Input: dimensioned drawing with shaded views. Units: mm. Origin: part minimum x, y, z. A direction names the side the tool comes from. Coordinates: 2 decimals unless noted, no trailing zeros. Write each loop counter-clockwise with the first axis right and the second up, starting at its lowest first coordinate (ties: lowest second). Pieces come first, ordered by that corner, then holes. Notation, with made-up numbers: (84.25, 32) -> (93.25, 32) arc R26 cw to (93.25, 56) -> close; hole circle Ø10 at (-19, 36). An arc over 180 degrees is marked (long way). One line per item, written item: value. Start each with the question number.
1. Access query for the marked faces 1 and 2. Directions: +Z, -Z, +X, -X, +Y, -Y. A direction counts if a zero-diameter tool reaches every point of the face in a straight line with its end or side. Return the directions, or none.
2. Section query C-C, the plane z = 3.75. Output: boundary loops of the cut face in (x, y), and give its area (3 significant figures).
3. Section query D-D, the plane y = 7. Output: boundary loops of the cut face in (x, z) (1 decimal).
4. First-contact query: P1, Ø3, axis at y = 3, z = 2, coming from the +X side; P2, Ø1, axis at y = 13, z = 8, coming from the +X side; P3, Ø3, axis at y = 10.5, z = 3, coming from the +X side (1 decimal); P4, Ø10, axis at x = 8.5, z = 14.5, coming from the +Y side. Flat tips, straight axial feed; report the tip coordinate or a pass-through.
5. Line query: line 1 (Z direction, x = 12, y = 14) (1 decimal); line 2 (Z direction, x = 9, y = 3.5) (1 decimal); line 3 (Y direction, x = 11, z = 27.5). Output: solid intervals per line, ascending.
6. Section query B-B, the plane z = 21.5. Output: boundary loops of the cut face in (x, y), and give its area (3 significant figures).
7. Section query A-A, the plane y = 20.32. Output: boundary loops of the cut face in (x, z) (1 decimal).
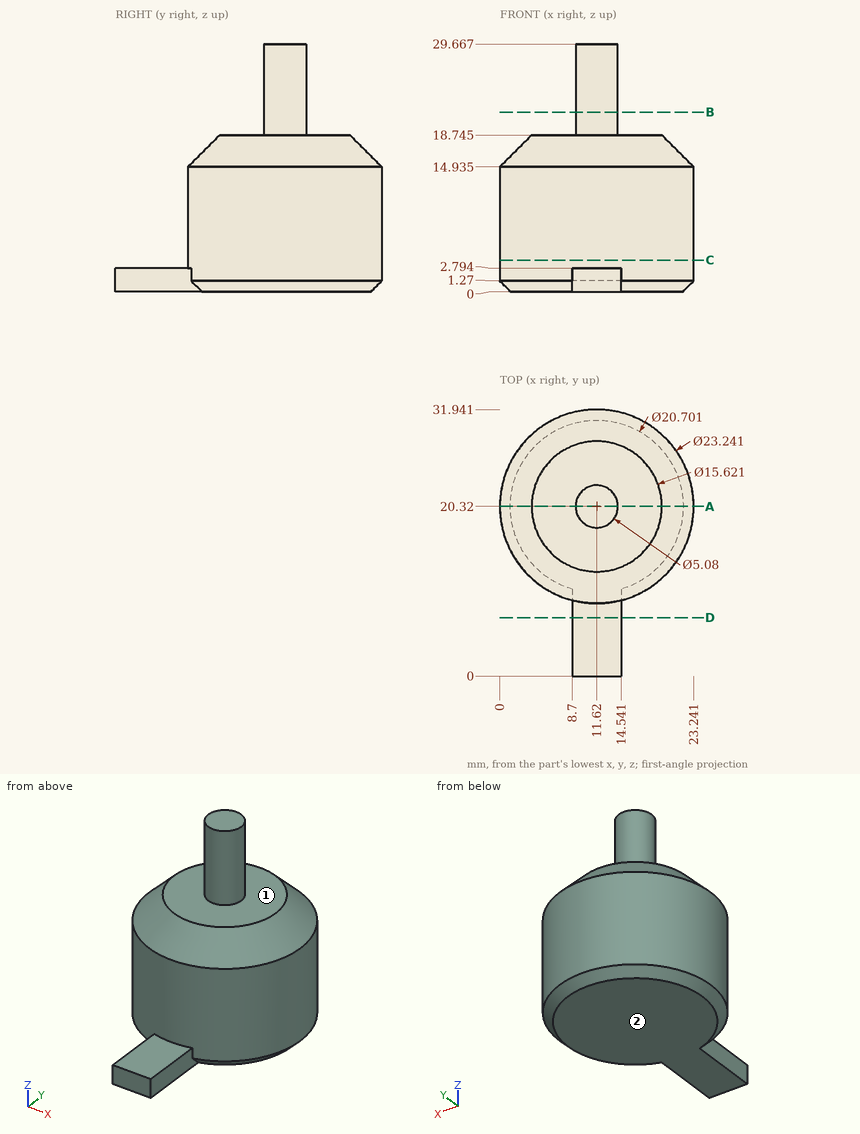
Computed values:
1. face 1: +Z
1. face 2: -Z, +X, -X, +Y, -Y
2. outline: circle Ø23.24 at (11.62, 20.32)
2. area: 424 mm²
3. outline: (8.7, 0) -> (14.5, 0) -> (14.5, 2.8) -> (8.7, 2.8) -> close
4. P1: stops at x = 14.54
4. P2: stops at x = 21.03
4. P3: stops at x = 19.7
4. P4: stops at y = 31.94
5. line 1: z = 0 to 18.7
5. line 2: z = 0 to 2.8
5. line 3: y = 17.86 to 22.78
6. outline: circle Ø5.08 at (11.62, 20.32)
6. area: 20.3 mm²
7. outline: (0, 1.3) -> (1.3, 0) -> (22, 0) -> (23.2, 1.3) -> (23.2, 14.9) -> (19.4, 18.7) -> (14.2, 18.7) -> (14.2, 29.7) -> (9.1, 29.7) -> (9.1, 18.7) -> (3.8, 18.7) -> (0, 14.9) -> close
